```python
from build123d import *

# Parameters (mm, degrees)
SKETCH_1_W      = 99
SKETCH_1_H      = 143
SKETCH_1_W_2    = 75
SKETCH_1_H_2    = 134
SKETCH_1_R      = 1.05
EXTRUDE_1_DEPTH = 1.6


with BuildPart() as part:
    # 草图1 → 凸台-拉伸1 (new body)
    with BuildSketch(Plane(origin=(0, 0, 0), x_dir=(1, 0, 0), z_dir=(0, 1, 0))):
        with Locations((49.5, -71.5)):
            Rectangle(SKETCH_1_W, SKETCH_1_H)
        with Locations((47, -71.5)):
            Rectangle(SKETCH_1_W_2, SKETCH_1_H_2, mode=Mode.SUBTRACT)
        with Locations(Location((94.8, -94.8, 0), (0, 0, 270))):
            Circle(SKETCH_1_R, mode=Mode.SUBTRACT)
        with Locations(Location((7, -7, 0), (0, 0, 270))):
            Circle(SKETCH_1_R, mode=Mode.SUBTRACT)
        with Locations(Location((96.3, -55.2, 0), (0, 0, 270))):
            Circle(SKETCH_1_R, mode=Mode.SUBTRACT)
        with Locations(Location((94.8, -26.8, 0), (0, 0, 270))):
            Circle(SKETCH_1_R, mode=Mode.SUBTRACT)
        with Locations(Location((87, -7, 0), (0, 0, 270))):
            Circle(SKETCH_1_R, mode=Mode.SUBTRACT)
        with Locations(Location((7, -136, 0), (0, 0, 270))):
            Circle(SKETCH_1_R, mode=Mode.SUBTRACT)
        with Locations(Location((87, -136, 0), (0, 0, 270))):
            Circle(SKETCH_1_R, mode=Mode.SUBTRACT)
    extrude(amount=EXTRUDE_1_DEPTH)


solid = part.part
```
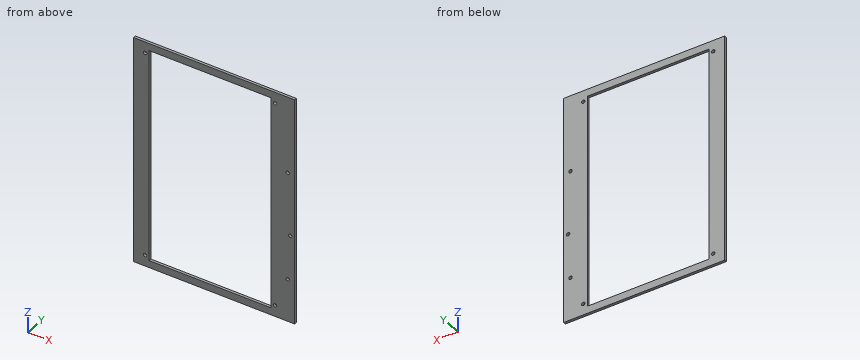
Model file for the job. Use its own axes, mm. Coordinates: 2 decimals unless noted, no trailing zeros. Write each loop counter-clockwise with the first axis right and the second up, starting at its lowest first coordinate (ties: lowest second). Pieces come first, ordered by that corner, then holes. Notation, with made-up numbers: (12, 80.25) - (66, 80.25) arc R15 ccw to (66, 98.25) - close; hole circle Ø3 at (49, 16.5). An arc over 180 degrees is marked (long way). One line per item, written item: value. Start each with the question number.
1. Flat gauge pin, fed straight in: pin 1 (1.3 mm diameter, centred on x = 87, z = 136, fed in from -Y). Where does the tip first touch, or does it go through?
2. Probe line 1 (X direction, y = 1.2, z = 26.8); line 2 (X direction, y = 1.1, z = 7); line 3 (Z direction, x = 94.8, y = 1.05). List the from-to ranges inside material, lowest first. Write a range as from..to.
3. Slice it at A-A (x = 49.5). Write the cut outline in (y, z), plus the area to 3 significant figures.
4. Slice it at B-B (z = 66.5). Write the cut outline in (x, y).
Answers below:
1. pin 1: passes through
2. line 1: x = 0..9.5, 84.5..93.75, 95.85..99
2. line 2: x = 0..5.95, 8.05..9.5, 84.5..85.95, 88.05..99
2. line 3: z = 0..25.75, 27.85..93.75, 95.85..143
3. outline: (0, 0) - (1.6, 0) - (1.6, 4.5) - (0, 4.5) - close; (0, 138.5) - (1.6, 138.5) - (1.6, 143) - (0, 143) - close
3. area: 14.4 mm^2
4. outline: (0, 0) - (9.5, 0) - (9.5, 1.6) - (0, 1.6) - close; (84.5, 0) - (99, 0) - (99, 1.6) - (84.5, 1.6) - close
